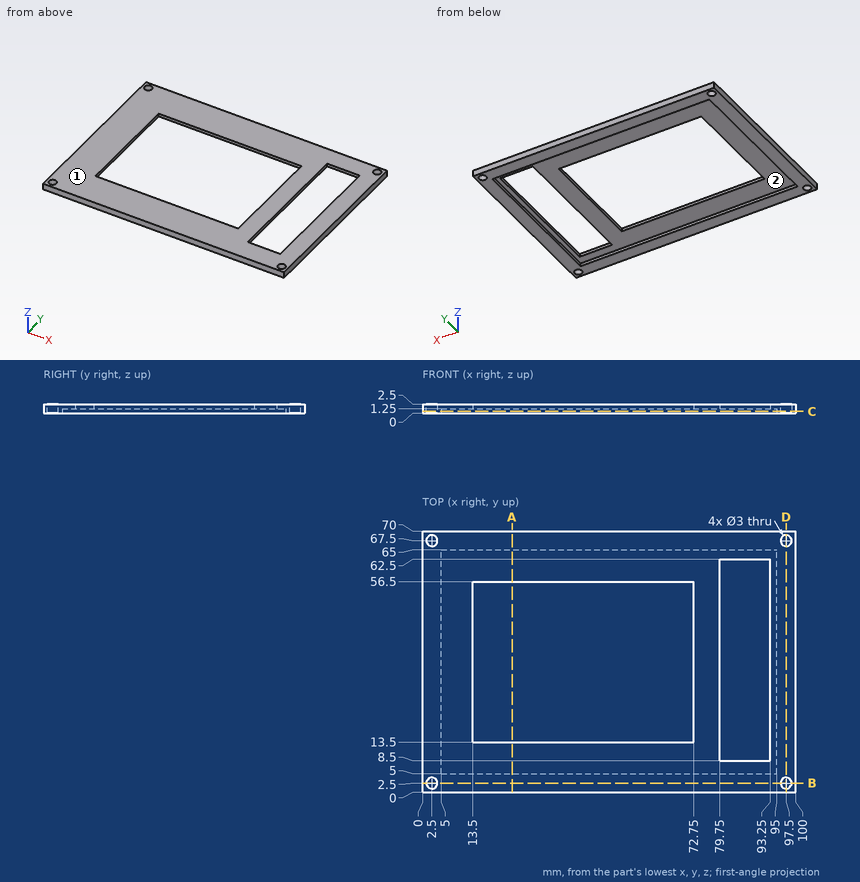
Verification items for this drawing (mm, ordinates from the low corner). Give positions to 0.01 mm unless a question says otherwise; leave off trailing zeros. Write each loop counter-clockwise with the first axis right and the second up, starting at its lowest first coordinate (ties: lowest second). Pieces come first, ordered by that corner, then holes.
1) Release check for a two-part mould opening along X. For the marked faces 1 and 2 record: released by +X, released by -X, zero draft, split by the parting line, or undercut.
Values follow:
face 1: zero draft
face 2: undercut
2) Go/stop test with a flat-tipped pin: pin 1 Ø2 at (x, y) = (37.5, 9.5) entering from -Z. Record where the tip stops, or that it passes through.
Values follow:
pin 1: stops at z = 1.25
3) Cross-section at D-D (x = 97.5). Record the boundary of the cut face in (y, z).
Values follow:
outline: (0, 0) - (1, 0) - (1, 2.5) - (0, 2.5) - close; (4, 0) - (66, 0) - (66, 2.5) - (4, 2.5) - close; (69, 0) - (70, 0) - (70, 2.5) - (69, 2.5) - close
4) Thickness scan on line 1 (X direction, y = 18, z = 1.9); line 2 (X direction, y = 67.5, z = 1.9); line 3 (Y direction, x = 2.5, z = 1.9). Record the ranges inside material, lowest first.
Values follow:
line 1: x = 0 to 13.5, 72.75 to 79.75, 93.25 to 100
line 2: x = 0 to 1, 4 to 96, 99 to 100
line 3: y = 0 to 1, 4 to 66, 69 to 70
5) Cross-section at A-A (x = 24). Record the boundary of the cut face in (y, z).
Values follow:
outline: (0, 0) - (5, 0) - (5, 1.25) - (13.5, 1.25) - (13.5, 2.5) - (0, 2.5) - close; (56.5, 1.25) - (65, 1.25) - (65, 0) - (70, 0) - (70, 2.5) - (56.5, 2.5) - close
6) Cross-section at C-C (z = 0.55). Record the boundary of the cut face in (x, y).
Values follow:
outline: (0, 0) - (100, 0) - (100, 70) - (0, 70) - close; hole circle Ø3 at (2.5, 2.5); hole circle Ø3 at (2.5, 67.5); hole (5, 5) - (95, 5) - (95, 65) - (5, 65) - close; hole circle Ø3 at (97.5, 2.5); hole circle Ø3 at (97.5, 67.5)
7) Cross-section at B-B (y = 2.5). Record the boundary of the cut face in (x, z).
Values follow:
outline: (0, 0) - (1, 0) - (1, 2.5) - (0, 2.5) - close; (4, 0) - (96, 0) - (96, 2.5) - (4, 2.5) - close; (99, 0) - (100, 0) - (100, 2.5) - (99, 2.5) - close
